Verification items for the finished model (mm, model axes). Face numbers are marked on the shaded views. A direction names the side the tool comes from. Round coordinates to 2 decimals unless told otherwise and drop trailing zeros. Write each loop counter-clockwise with the first axis right and the second up, starting at its lowest first coordinate (ties: lowest second). Pieces come first, ordered by that corner, then holes. Notation, with made-up numbers: (34, -8) - (83, -8) arc R25 ccw to (83, 7) - close; hole circle Ø4 at (19.25, -28). An arc over 180 degrees is marked (long way). Answer as a JSON object with one key per item and string values. Group by question number.
1) Mould release check, pull along Y, two halves, no side actions. Record for the marked faces 1, 2 and 3: +Y half, -Y half, draft (parallel to the pull), parting line (faces both ways), or undercut.
2) Section check A-A (y = 0). Enter the section's corners in (x, z), then the cut area to 3 significant figures.
3) Go/stop test with flat-tipped pins: pin 1 Ø3.5 at (y, z) = (-26.526, 5) entering from +X; pin 2 Ø3 at (y, z) = (60, 5) entering from +X; pin 3 Ø4 at (x, y) = (-5.5, -27.5) entering from +Z. Record where each tip stops, or that it passes through.
4) Thickness scan on line 1 (Y direction, x = -45.5, z = 5) (1 decimal); line 2 (X direction, y = -24, z = 1); line 3 (X direction, y = 0, z = 1). Record the ranges inside material, lowest first.
5) Set-up check for the marked faces 4 and 5: record each of +Z, -Z, +X, -X, +Y, -Y from which the full face is reachable in a straight line by a thin tool's end or side.
6) Section check D-D (x = 31). Enter the section's corners in (y, z), then the cut area to 3 significant figures.
7) Section check B-B (x = 3.5). Enter the section's corners in (y, z).
8) Section check C-C (z = 1.5). Enter the section's corners in (x, y), then the cut area to 3 significant figures.
Autodesk Inventor part; units mm, degrees
ref_plane "Work Plane1" through (0, 0, 0) normal (0, 0, 1) x (1, 0, 0)
ref_plane "YZ Plane" through (0, 0, 0) normal (1, 0, 0) x (0, 1, 0)
ref_plane "XZ Plane" through (0, 0, 0) normal (0, 1, 0) x (-1, 0, 0)
ref_plane "Work Plane1" through (0, 0, 0) normal (0, 0, 1) x (1, 0, 0)
sketch "Sketch1" plane through (0, 0, 0) normal (0, 0, 1) x (1, 0, 0)
  circle A0 centre (0, 0) radius 21
  circle A1 centre (23.57, -23.57) radius 2
  circle A2 centre (23.57, 23.57) radius 2
  circle A3 centre (-23.57, -23.57) radius 2.5
  circle A4 centre (-23.57, 23.57) radius 2
  circle A5 centre (-23.57, -23.57) radius 2
  circle A6 centre (0, 0) radius 19
  circle A7 centre (-23.57, 23.57) radius 2.5
  circle A8 centre (-23.57, -23.57) radius 2.5
  arc A9 (-29.95, -24.95) -> (-24.95, -29.95) centre (-24.95, -24.95) ccw
  line L0 (24.95, -29.95) -> (-24.95, -29.95)
  arc A10 (24.95, -29.95) -> (29.95, -24.95) centre (24.95, -24.95) ccw
  line L1 (29.95, 24.95) -> (29.95, -24.95)
  arc A11 (29.95, 24.95) -> (24.95, 29.95) centre (24.95, 24.95) ccw
  line L2 (-24.95, 29.95) -> (24.95, 29.95)
  arc A12 (-24.95, 29.95) -> (-29.95, 24.95) centre (-24.95, 24.95) ccw
  line L3 (-29.95, -24.95) -> (-29.95, 24.95)
  circle A13 centre (23.57, -23.57) radius 2.5
  circle A14 centre (23.57, 23.57) radius 2.5
  line L4 (-49.95, -90) -> (-49.95, 90)
  line L5 (-59.95, -90) -> (-49.95, -90)
  line L6 (-59.95, 90) -> (-49.95, 90)
  line L7 (40.2846, 0) -> (-40.2846, 0)
  line L8 (-49.95, -90) -> (-49.95, 90)
  line L9 (-59.95, -90) -> (-49.95, -90)
  line L10 (-49.95, 35.5095) -> (-26.95, 35.5095)
  line L11 (-24.95, 29.95) -> (-49.95, 29.95)
  line L12 (-24.95, -29.95) -> (-49.95, -29.95)
  circle A15 centre (0, 0) radius 22
  line L13 (-32.95, 22) -> (-32.95, -22)
  line L14 (-30.95, -14.95) -> (-49.95, -14.95)
  line L15 (-30.95, 14.95) -> (-49.95, 14.95)
  line L16 (-30.95, -14.95) -> (-30.95, 14.95)
  line L17 (24.7214, -34.026) -> (0, -42.0585)
  line L18 (0, -42.0585) -> (-24.7214, -34.026)
  line L19 (-24.7214, -34.026) -> (-40, -12.9968)
  line L20 (-40, -12.9968) -> (-40, 12.9968)
  line L21 (-40, 12.9968) -> (-24.7214, 34.026)
  line L22 (-24.7214, 34.026) -> (0, 42.0585)
  line L23 (0, 42.0585) -> (24.7214, 34.026)
  line L24 (24.7214, 34.026) -> (40, 12.9968)
  line L25 (40, 12.9968) -> (40, -12.9968)
  line L26 (40, -12.9968) -> (24.7214, -34.026)
  line L27 (-24.7214, -34.026) -> (-49.95, -34.026)
  line L28 (-24.7214, 34.026) -> (-49.95, 34.026)
  arc A16 (-24.7214, -34.026) -> (-24.7214, 34.026) centre (0, 0) ccw
  line L29 (-24.7214, 34.026) -> (-27.8, 34.026)
  line L30 (-27.8, 34.026) -> (-27.8, 80.5095)
  line L31 (-27.8, 80.5095) -> (-49.95, 80.5095)
  line L32 (-49.95, 80.5095) -> (-49.95, 14.95)
  line L33 (-49.95, 14.95) -> (-35.95, 14.95)
  arc A17 (-30.95, 9.95) -> (-35.95, 14.95) centre (-35.95, 9.95) ccw
  line L34 (-30.95, 9.95) -> (-30.95, -9.95)
  arc A18 (-35.95, -14.95) -> (-30.95, -9.95) centre (-35.95, -9.95) ccw
  line L35 (-35.95, -14.95) -> (-49.95, -14.95)
  line L36 (-49.95, -14.95) -> (-49.95, -34.026)
  line L37 (-49.95, -34.026) -> (-24.7214, -34.026)
  circle A19 centre (15.9909, -0.539) radius 1.6
  circle A20 centre (-11.6884, -10.9261) radius 2
  circle A21 centre (11.6884, 10.9261) radius 2
  circle A22 centre (10.9261, -11.6884) radius 2
  circle A23 centre (-15.9909, 0.539) radius 1.6
  circle A24 centre (-0.539, -15.9909) radius 1.6
  circle A25 centre (0, 0) radius 12.5
  circle A26 centre (0.539, 15.9909) radius 1.6
  circle A27 centre (-10.9261, 11.6884) radius 2
  point P0 (0, 0)
  point P1 (-23.2856, -45.1645)
  point P2 (-49.95, -75.9684)
  point P3 (-23.2856, 45.1645)
  point P4 (-49.95, -14.95)
  point P5 (-32.95, 13.95)
  point P6 (-32.95, 14.95)
  dimension "d9" = 1
  dimension "d10" = 15
  dimension "d11" = 15
  dimension "d12" = 1
  dimension "d13" = 40
extrude "Extrusion1" add sketch "Sketch1" along normal blind 10 contours L7 A15 A0 | A0 L7 A15 | A15 L7 L3 A12 L2 A11 L1 | L7 L1 A10 L0 A9 L3 A15 | L7 L25 L26 L17 L18 L19 L12 L0 A10 L1 | L1 A11 L2 L11 L21 L22 L23 L24 L25 L7 | L7 L16 L15 L21 L11 A12 L3 | L3 A9 L12 L19 L14 L16 L7 | L25 A16 | L16 A18 L13 L7 | L7 L13 A17 L16 | L24 A16 | A16 L26 | L13 A18 L14 L19 L20 L7 | L7 L20 L21 L15 A17 L13 | L16 L14 L13 A18 | A17 L13 L15 L16 | L23 A16 | A16 L17 | L19 L27 L4 L12 | L12 L4 L14 L19 | L21 L15 L4 L11 | L11 L4 L28 L21 | L20 L19 L14 L4 L15 L21 | A17 L15 L13 | L13 L14 A18 | L22 A16 | A16 L18 | A1 | A2 | A3 | A4 | A5 | A7 | A13 | A14
sketch "Sketch2" plane through (-49.95, -34.026, 0) normal (-1, 0, 0) x (0, 0, 1)
  line L0 (0, 68.0521) -> (0, 0)
  line L1 (0, 0) -> (10, 0)
  line L2 (10, 68.0521) -> (10, 0)
  line L3 (0, 68.0521) -> (0, 0)
  line L4 (10, 68.0521) -> (10, 0)
  line L5 (0, 68.0521) -> (10, 68.0521)
  line L6 (0, 0) -> (10, 0)
  line L7 (0, 68.0521) -> (10, 68.0521)
  point P0 (0, 34.026)
  point P1 (5, 7.5)
  point P2 (5, 60.5521)
  point P3 (5, 68.0521)
  point P4 (5, 19.076)
  dimension "d24" = 7.5
  dimension "d25" = 7.5
hole "Hole1" at (-49.95, 26.526, 5) at (-49.95, -26.526, 5) direction (1, 0, 0) diameter 3.242 depth 15 tip angle 118
sketch "Sketch3" plane through (0, 0, 10) normal (0, 0, 1) x (1, 0, 0)
  arc A0 (-24.7214, -34.026) -> (-24.7214, 34.026) centre (0, 0) ccw
  line L0 (-24.7214, 34.026) -> (-27.8, 34.026)
  line L1 (-27.8, 34.026) -> (-27.8, 80.5095)
  line L2 (-27.8, 80.5095) -> (-49.95, 80.5095)
  line L3 (-49.95, 80.5095) -> (-49.95, 14.95)
  line L4 (-49.95, 14.95) -> (-35.95, 14.95)
  arc A1 (-30.95, 9.95) -> (-35.95, 14.95) centre (-35.95, 9.95) ccw
  line L5 (-30.95, 9.95) -> (-30.95, -9.95)
  arc A2 (-35.95, -14.95) -> (-30.95, -9.95) centre (-35.95, -9.95) ccw
  line L6 (-35.95, -14.95) -> (-49.95, -14.95)
  line L7 (-49.95, -14.95) -> (-49.95, -34.026)
  line L8 (-49.95, -34.026) -> (-24.7214, -34.026)
  circle A3 centre (15.9909, -0.539) radius 1.6
  circle A4 centre (-11.6884, -10.9261) radius 2
  circle A5 centre (11.6884, 10.9261) radius 2
  circle A6 centre (10.9261, -11.6884) radius 2
  circle A7 centre (-15.9909, 0.539) radius 1.6
  circle A8 centre (-0.539, -15.9909) radius 1.6
  circle A9 centre (0, 0) radius 12.5
  circle A10 centre (0.539, 15.9909) radius 1.6
  circle A11 centre (-10.9261, 11.6884) radius 2
  circle A12 centre (0, 0) radius 19
  circle A13 centre (-23.57, 23.57) radius 2.5
  circle A14 centre (-23.57, -23.57) radius 2.5
  arc A15 (-29.95, -24.95) -> (-24.95, -29.95) centre (-24.95, -24.95) ccw
  line L9 (24.95, -29.95) -> (-24.95, -29.95)
  arc A16 (24.95, -29.95) -> (29.95, -24.95) centre (24.95, -24.95) ccw
  line L10 (29.95, 24.95) -> (29.95, -24.95)
  arc A17 (29.95, 24.95) -> (24.95, 29.95) centre (24.95, 24.95) ccw
  line L11 (-24.95, 29.95) -> (24.95, 29.95)
  arc A18 (-24.95, 29.95) -> (-29.95, 24.95) centre (-24.95, 24.95) ccw
  line L12 (-29.95, -24.95) -> (-29.95, 24.95)
  circle A19 centre (23.57, -23.57) radius 2.5
  circle A20 centre (23.57, 23.57) radius 2.5
  arc A21 (-37.4079, -14.95) -> (-37.4079, 14.95) centre (0, 0) ccw
  line L13 (-27.8, 34.026) -> (-27.8, 29.155)
  line L14 (-49.95, -34.026) -> (-21.5657, -34.026)
  line L15 (-49.95, -34.026) -> (-24.7214, -34.026)
  point P0 (0, 0)
  point P1 (-24.7214, -34.026)
extrude "Extrusion2" cut sketch "Sketch3" against normal blind 10 contours L14 A21 L13 L0 A0
sketch "Sketch4" plane through (0, 0, 10) normal (0, 0, 1) x (1, 0, 0)
  arc A0 (-24.7214, -34.026) -> (-24.7214, 34.026) centre (0, 0) ccw
  line L0 (-24.7214, 34.026) -> (-27.8, 34.026)
  line L1 (-27.8, 34.026) -> (-27.8, 80.5095)
  line L2 (-27.8, 80.5095) -> (-49.95, 80.5095)
  line L3 (-49.95, 80.5095) -> (-49.95, 14.95)
  line L4 (-49.95, 14.95) -> (-35.95, 14.95)
  arc A1 (-30.95, 9.95) -> (-35.95, 14.95) centre (-35.95, 9.95) ccw
  line L5 (-30.95, 9.95) -> (-30.95, -9.95)
  arc A2 (-35.95, -14.95) -> (-30.95, -9.95) centre (-35.95, -9.95) ccw
  line L6 (-35.95, -14.95) -> (-49.95, -14.95)
  line L7 (-49.95, -14.95) -> (-49.95, -34.026)
  line L8 (-49.95, -34.026) -> (-24.7214, -34.026)
  circle A3 centre (15.9909, -0.539) radius 1.6
  circle A4 centre (-11.6884, -10.9261) radius 2
  circle A5 centre (11.6884, 10.9261) radius 2
  circle A6 centre (10.9261, -11.6884) radius 2
  circle A7 centre (-15.9909, 0.539) radius 1.6
  circle A8 centre (-0.539, -15.9909) radius 1.6
  circle A9 centre (0, 0) radius 12.5
  circle A10 centre (0.539, 15.9909) radius 1.6
  circle A11 centre (-10.9261, 11.6884) radius 2
  line L9 (-49.95, -90) -> (-49.95, 90)
  line L10 (-59.95, 90) -> (-49.95, 90)
  line L11 (-49.95, -90) -> (-49.95, 90)
  line L12 (-27.8, 29.155) -> (-27.8, 34.026)
  line L13 (-27.8, 34.026) -> (-49.95, 34.026)
  line L14 (-49.95, 34.026) -> (-49.95, -34.026)
  line L15 (-49.95, -34.026) -> (-21.5657, -34.026)
  arc A12 (-21.5657, -34.026) -> (-27.8, 29.155) centre (0, 0) ccw
  circle A13 centre (0, 0) radius 21
  point P0 (0, 0)
extrude "Extrusion3" add sketch "Sketch4" against normal blind 10 contours L13 L3 L2 L1
fillet "Fillet1" radius 2 2 edges at (-27.8, 29.155, 5) (-21.5657, -34.026, 5)
fillet "Fillet2" radius 1 1 edges at (-27.8, 80.5095, 5)
sketch "Sketch5" plane through (-27.8, 33.5015, 10) normal (1, 0, 0) x (0, 0, -1)
  arc A0 (8, 9.19) -> (10, 11.19) centre (8, 11.19) ccw
  line L0 (10, 49.19) -> (10, 11.19)
  arc A1 (10, 49.19) -> (8, 51.19) centre (8, 49.19) ccw
  line L1 (-60.5, 51.19) -> (8, 51.19)
  arc A2 (-60.5, 51.19) -> (-62.5, 49.19) centre (-60.5, 49.19) ccw
  line L2 (-62.5, 11.19) -> (-62.5, 49.19)
  arc A3 (-62.5, 11.19) -> (-60.5, 9.19) centre (-60.5, 11.19) ccw
  line L3 (8, 9.19) -> (-60.5, 9.19)
  circle A4 centre (-26.25, 30.19) radius 12.6
  circle A5 centre (-26.25, 14.19) radius 2
  arc A6 (-59.6, 14.79) -> (-55.4, 14.79) centre (-57.5, 14.79) ccw
  line L4 (-59.6, 45.59) -> (-59.6, 14.79)
  arc A7 (-55.4, 45.59) -> (-59.6, 45.59) centre (-57.5, 45.59) ccw
  line L5 (-55.4, 14.79) -> (-55.4, 45.59)
  circle A8 centre (-42.25, 30.19) radius 2
  circle A9 centre (-37.5637, 18.8763) radius 1.5
  circle A10 centre (-37.5637, 41.5037) radius 1.5
  circle A11 centre (-14.9363, 18.8763) radius 1.5
  arc A12 (7.1, 45.59) -> (2.9, 45.59) centre (5, 45.59) ccw
  line L6 (7.1, 14.79) -> (7.1, 45.59)
  arc A13 (2.9, 14.79) -> (7.1, 14.79) centre (5, 14.79) ccw
  line L7 (2.9, 45.59) -> (2.9, 14.79)
  circle A14 centre (-10.25, 30.19) radius 2
  circle A15 centre (-14.9363, 41.5037) radius 1.5
  circle A16 centre (-26.25, 46.19) radius 2
  circle A17 centre (-57.5, 11.46) radius 1.621
  circle A18 centre (-57.5, 26.86) radius 1.621
  arc A19 (8, 9.19) -> (10, 11.19) centre (8, 11.19) ccw
  line L8 (10, 49.19) -> (10, 11.19)
  arc A20 (10, 49.19) -> (8, 51.19) centre (8, 49.19) ccw
  line L9 (-60.5, 51.19) -> (8, 51.19)
  arc A21 (-60.5, 51.19) -> (-62.5, 49.19) centre (-60.5, 49.19) ccw
  line L10 (-62.5, 11.19) -> (-62.5, 49.19)
  arc A22 (-62.5, 11.19) -> (-60.5, 9.19) centre (-60.5, 11.19) ccw
  line L11 (8, 9.19) -> (-60.5, 9.19)
  circle A23 centre (-26.25, 30.19) radius 12.6
  circle A24 centre (-26.25, 14.19) radius 2
  arc A25 (-59.6, 14.79) -> (-55.4, 14.79) centre (-57.5, 14.79) ccw
  line L12 (-59.6, 45.59) -> (-59.6, 14.79)
  arc A26 (-55.4, 45.59) -> (-59.6, 45.59) centre (-57.5, 45.59) ccw
  line L13 (-55.4, 14.79) -> (-55.4, 45.59)
  circle A27 centre (-42.25, 30.19) radius 2
  circle A28 centre (-37.5637, 18.8763) radius 1.5
  circle A29 centre (-37.5637, 41.5037) radius 1.5
  circle A30 centre (-14.9363, 18.8763) radius 1.5
  arc A31 (7.1, 45.59) -> (2.9, 45.59) centre (5, 45.59) ccw
  line L14 (7.1, 14.79) -> (7.1, 45.59)
  arc A32 (2.9, 14.79) -> (7.1, 14.79) centre (5, 14.79) ccw
  line L15 (2.9, 45.59) -> (2.9, 14.79)
  circle A33 centre (-10.25, 30.19) radius 2
  circle A34 centre (-14.9363, 41.5037) radius 1.5
  circle A35 centre (-26.25, 46.19) radius 2
  arc A36 (8, 9.19) -> (10, 11.19) centre (8, 11.19) ccw
  line L16 (10, 49.19) -> (10, 11.19)
  arc A37 (10, 49.19) -> (8, 51.19) centre (8, 49.19) ccw
  line L17 (-60.5, 51.19) -> (8, 51.19)
  arc A38 (-60.5, 51.19) -> (-62.5, 49.19) centre (-60.5, 49.19) ccw
  line L18 (-62.5, 11.19) -> (-62.5, 49.19)
  arc A39 (-62.5, 11.19) -> (-60.5, 9.19) centre (-60.5, 11.19) ccw
  line L19 (8, 9.19) -> (-60.5, 9.19)
  circle A40 centre (-26.25, 30.19) radius 12.6
  circle A41 centre (-26.25, 14.19) radius 2
  arc A42 (-59.6, 14.79) -> (-55.4, 14.79) centre (-57.5, 14.79) ccw
  line L20 (-59.6, 45.59) -> (-59.6, 14.79)
  arc A43 (-55.4, 45.59) -> (-59.6, 45.59) centre (-57.5, 45.59) ccw
  line L21 (-55.4, 14.79) -> (-55.4, 45.59)
  circle A44 centre (-42.25, 30.19) radius 2
  circle A45 centre (-37.5637, 18.8763) radius 1.5
  circle A46 centre (-37.5637, 41.5037) radius 1.5
  circle A47 centre (-14.9363, 18.8763) radius 1.5
  arc A48 (7.1, 45.59) -> (2.9, 45.59) centre (5, 45.59) ccw
  line L22 (7.1, 14.79) -> (7.1, 45.59)
  arc A49 (2.9, 14.79) -> (7.1, 14.79) centre (5, 14.79) ccw
  line L23 (2.9, 45.59) -> (2.9, 14.79)
  circle A50 centre (-10.25, 30.19) radius 2
  circle A51 centre (-14.9363, 41.5037) radius 1.5
  circle A52 centre (-26.25, 46.19) radius 2
  point P0 (10, -33.5015)
  point P1 (5, 22.29)
  point P2 (5, 38.09)
  dimension "d47" = 7.5
  dimension "d48" = 7.5
hole "Hole2" at (-27.8, 55.7915, 5) at (-27.8, 71.5915, 5) direction (-1, 0, 0) diameter 3.242 depth 22.15
sketch "Sketch7" plane through (0, 0, 10) normal (0, 0, 1) x (1, 0, 0)
  circle A0 centre (0, 0) radius 32.75
  dimension "d49" = 65.5
extrude "Extrusion5" cut sketch "Sketch7" against normal blind 7
sketch "Sketch10" plane through (0, 0, 0) normal (0, 0, -1) x (-1, 0, 0)
  point P0 (0, 0)
  point P1 (-23.57, -23.57)
  point P2 (-23.57, 23.57)
  point P3 (23.57, 23.57)
  point P4 (23.57, -23.57)
hole "Hole3" at (23.57, -23.57, 0) at (23.57, 23.57, 0) at (-23.57, 23.57, 0) at (-23.57, -23.57, 0) direction (0, 0, 1) diameter 3.242 depth 12 tip angle 118
equation "\"d11\" = d10"
properties part number "base frame achterkant 10 mm" material "Aluminum 6061"
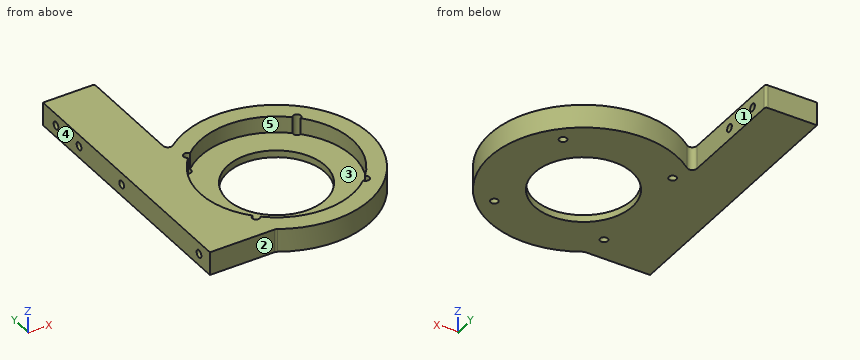
Returned:
{
 "1": {"face 1": "draft", "face 2": "-Y half", "face 3": "undercut"},
 "2": {"outline": "(-49.95, 0) - (-21, 0) - (-21, 3) - (-32.75, 3) - (-32.75, 10) - (-49.95, 10) - close; (21, 0) - (40.28, 0) - (40.28, 10) - (32.75, 10) - (32.75, 3) - (21, 3) - close", "area": "318 mm2"},
 "3": {"pin 1": "x = 31.76", "pin 2": "x = -27.8", "pin 3": "z = 3"},
 "4": {"line 1": "-34 to -28.1, -24.9 to 24.9, 28.1 to 54.2, 57.4 to 70, 73.2 to 80.5", "line 2": "-49.95 to -25.13, -22.01 to 22.01, 25.13 to 32.36", "line 3": "-49.95 to -21, 21 to 40.28"},
 "5": {"face 4": "+Z, -Z, -X, +Y, -Y", "face 5": "+Z"},
 "6": {"outline": "(-25.73, 0) - (25.73, 0) - (25.73, 10) - (10.56, 10) - (10.56, 3) - (-10.56, 3) - (-10.56, 10) - (-25.73, 10) - close", "area": "367 mm2"},
 "7": {"outline": "(-40.13, 0) - (-20.71, 0) - (-20.71, 3) - (-32.56, 3) - (-32.56, 10) - (-40.13, 10) - close; (20.71, 0) - (40.13, 0) - (40.13, 10) - (32.56, 10) - (32.56, 3) - (20.71, 3) - close"},
 "8": {"outline": "(-49.95, -34.03) - (-22.14, -34.03) arc R2 cw to (-21.09, -34.32) arc R40.28 ccw (long way) to (-24.58, 31.92) arc R2 cw to (-27.8, 33.5) - (-27.8, 79.51) arc R1 ccw to (-28.8, 80.51) - (-49.95, 80.51) - close; hole circle Ø3.24 at (-23.57, -23.57); hole circle Ø3.24 at (-23.57, 23.57); hole circle Ø42 at (0, 0); hole circle Ø3.24 at (23.57, -23.57); hole circle Ø3.24 at (23.57, 23.57)", "area": "5,730 mm2"}
}
